The drawing under review shows one solid part. Ordinate dimensions are in mm from its lowest x, y, z. A direction names the side the tool comes from. Coordinates: 2 decimals unless noted, no trailing zeros. Order: outer loops, then holes, each group sorted by start corner. A loop starts at its lowest first (then second) coordinate and runs counter-clockwise, first axis right, second up. Notation, with made-up numbers: (-17.5, -29) -> (28.5, -29) arc R20 cw to (28.5, 3) -> close; hole circle Ø2 at (55.5, -30.5). An arc over 180 degrees is marked (long way). Put each result on its own line as item: value.
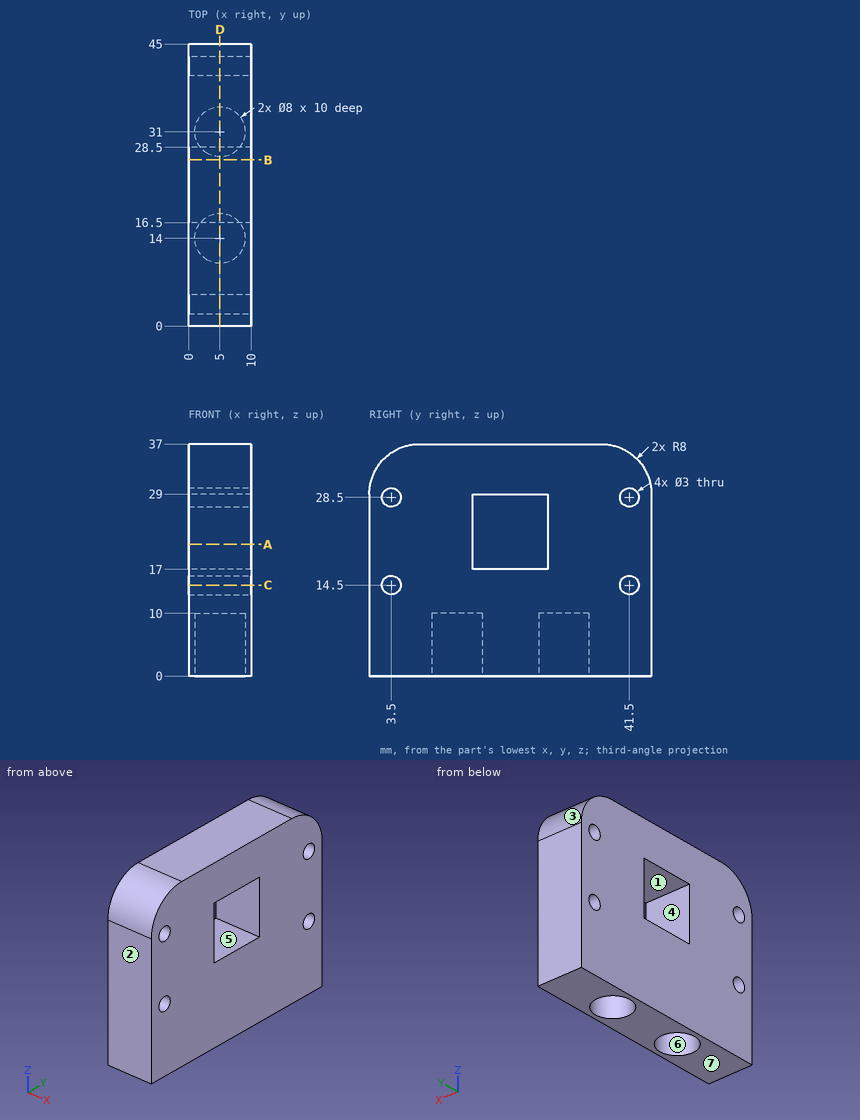
Item 1: Consider section C-C on z = 14.5. Write out the cut boundary in (x, y), and give its area (3 significant figures).
Answers below:
outline: (0, 0) -> (10, 0) -> (10, 2) -> (0, 2) -> close; (0, 5) -> (10, 5) -> (10, 40) -> (0, 40) -> close; (0, 43) -> (10, 43) -> (10, 45) -> (0, 45) -> close
area: 390 mm^2
Item 2: Consider section D-D on x = 5. Write out the cut boundary in (y, z), and give its area (3 significant figures).
Answers below:
outline: (0, 0) -> (10, 0) -> (10, 10) -> (18, 10) -> (18, 0) -> (27, 0) -> (27, 10) -> (35, 10) -> (35, 0) -> (45, 0) -> (45, 29) arc R8 ccw to (37, 37) -> (8, 37) arc R8 ccw to (0, 29) -> close; hole circle Ø3 at (3.5, 14.5); hole circle Ø3 at (3.5, 28.5); hole (16.5, 17) -> (28.5, 17) -> (28.5, 29) -> (16.5, 29) -> close; hole circle Ø3 at (41.5, 14.5); hole circle Ø3 at (41.5, 28.5)
area: 1,310 mm^2
Item 3: For the marked faces 5, 6 and 7, list the 3-axis set-ups (+Z, -Z, +X, -X, +Y, -Y) from which the entire face can be reached by the end or side of a thin tool; tool diameter is ignored.
Answers below:
face 5: +X, -X
face 6: -Z
face 7: -Z, +X, -X, +Y, -Y
Item 4: Mouldability with a two-part tool opening along Y and no side actions: class the marked faces 1, 2, 3 and 4 as +Y half, -Y half, draft (parallel to the pull), parting line (faces both ways), or undercut.
Answers below:
face 1: undercut
face 2: -Y half
face 3: +Y half
face 4: undercut
Item 5: Consider section B-B on y = 26.5. Write out the cut boundary in (x, z).
Answers below:
outline: (0, 0) -> (10, 0) -> (10, 17) -> (0, 17) -> close; (0, 29) -> (10, 29) -> (10, 37) -> (0, 37) -> close
Item 6: For pin 1 Ø2.5 at (y, z) = (3.5, 28.5) entering from -X; pin 2 Ø5 at (x, y) = (8.5, 36) entering from -Z, all flat-tipped, find the tip position at first contact; note any pin that passes through.
Answers below:
pin 1: through
pin 2: z = 0
Item 7: For line 1 (Y direction, x = 5, z = 6); line 2 (Y direction, x = 2.75, z = 14.5); line 3 (Y direction, x = 3, z = 28.5), list the stretches that pass through material, from the lowest coordinate up. Write a range as from..to.
Answers below:
line 1: 0..10, 18..27, 35..45
line 2: 0..2, 5..40, 43..45
line 3: 0..2, 5..16.5, 28.5..40, 43..45
Item 8: Consider section A-A on z = 21. Write out the cut boundary in (x, y), and give its area (3 significant figures).
Answers below:
outline: (0, 0) -> (10, 0) -> (10, 16.5) -> (0, 16.5) -> close; (0, 28.5) -> (10, 28.5) -> (10, 45) -> (0, 45) -> close
area: 330 mm^2
